Verification items for this drawing (mm, ordinates from the low corner). Coordinates: 2 decimals unless noted, no trailing zeros. Loops run counter-clockwise (first coordinate to the right, second up) from the corner with the lowest first, then second, coordinate; pieces in that order, holes last. Notation, with made-up numbers: (-21, -33.75) -> (18, -33.75) arc R25 ccw to (18, -19.75) -> close; hole circle Ø4 at (20.25, -25). An arc over 180 degrees is marked (long way). Write item = value, one per line.
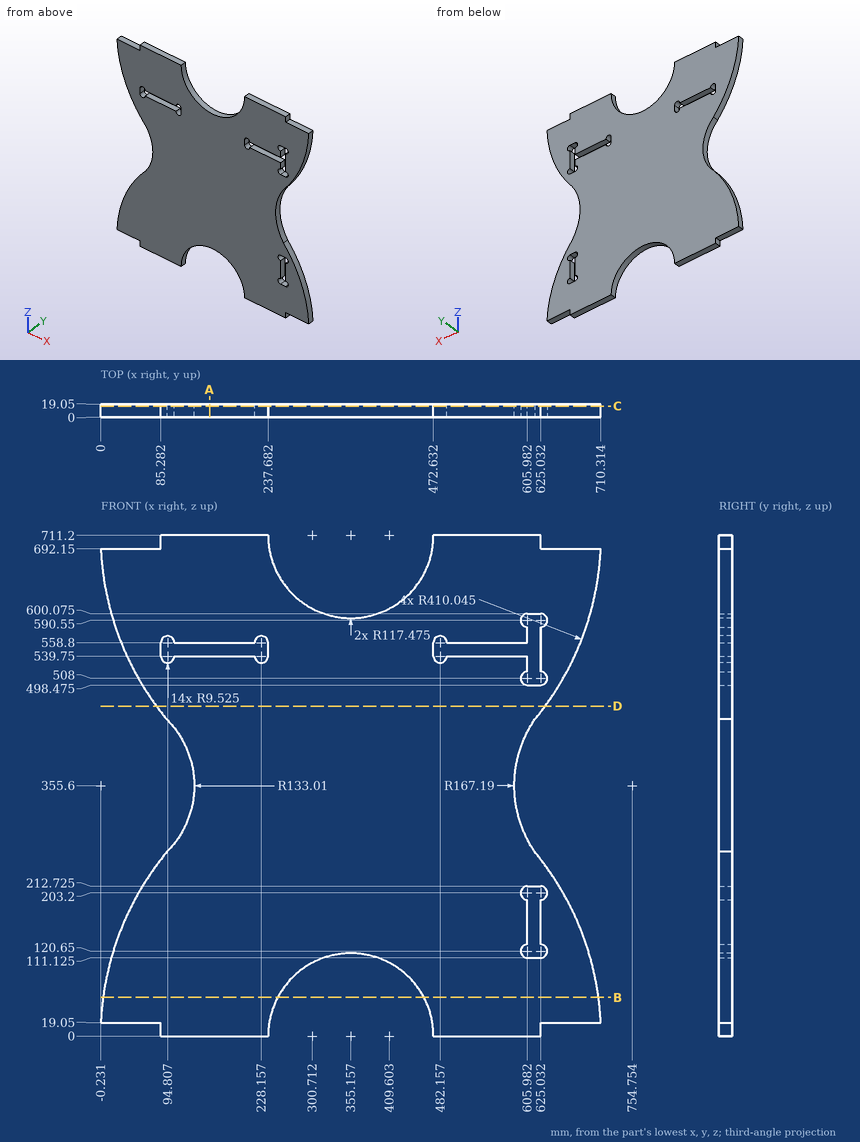
1) Sectioned sample at C-C, the plane y = 16. Count the separate pieces of the cut face and the enclosed holes in it, plus the area to 3 significant figures.
Ans:
separate_pieces = 1
enclosed_holes = 3
area = 369,000 mm2
2) Material ranges on line 1 (Z direction, x = 184, y = 2); line 2 (X direction, y = 16, z = 537) (1 decimal); line 3 (X direction, y = 17.5, z = 450) (1 decimal), recorded low to high.
Ans:
line_1 = 0 to 539.75, 558.8 to 711.2
line_2 = 38.4 to 85.7, 103.9 to 219, 237.3 to 473, 491.3 to 606, 625 to 671.9
line_3 = 93.5 to 616.8
3) Depth check by flat-ended pin: pin 1 Ø5 at (y, z) = (8.5, 368) entering from -X; pin 2 Ø9.5 at (y, z) = (11, 550.5) entering from +X; pin 3 Ø5.5 at (x, y) = (646.5, 13) entering from -Z. Enter the tip coordinate at first touch or a pass-through.
Ans:
pin_1 = 131.94
pin_2 = 679.94
pin_3 = 19.05
4) Sectioned sample at B-B, the plane z = 55. Record the cut outline in (x, y), plus the area to 3 significant figures.
Ans:
outline = (3.26, 0) -> (251.35, 0) -> (251.35, 19.05) -> (3.26, 19.05) -> close; (458.96, 0) -> (707.05, 0) -> (707.05, 19.05) -> (458.96, 19.05) -> close
area = 9,450 mm2
5) Sectioned sample at A-A, the plane x = 154.5. Record the cut outline in (y, z).
Ans:
outline = (0, 0) -> (19.05, 0) -> (19.05, 539.75) -> (0, 539.75) -> close; (0, 558.8) -> (19.05, 558.8) -> (19.05, 711.2) -> (0, 711.2) -> close
6) Sectioned sample at D-D, the plane z = 468.5. Record the cut outline in (x, y), plus the area to 3 significant figures.
Ans:
outline = (79.1, 0) -> (631.22, 0) -> (631.22, 19.05) -> (79.1, 19.05) -> close
area = 10,500 mm2
